Part model, mm, in its own coordinate system. A direction names the side the tool comes from. Round coordinates to 2 decimals unless told otherwise and drop trailing zeros. Write each loop counter-clockwise with the first axis right and the second up, starting at its lowest first coordinate (ties: lowest second). Pieces come first, ordered by that corner, then holes. Notation, with made-up numbers: M 26,72.5 L 42,72.5 A22 cw 42,96.5 Z; hole C 33.25,-37.75 d10. An arc over 180 degrees is marked long. Use a Markdown table: item, result. Add a question column.
1) Slice it at B-B on x = -7.5. Write the cut outline in (y, z), plus the area to 3 significant figures.
2) Two-plate mould, pull along Y, no slides. Class faces 1 (the face through (0, 2, -1)), 2 (the face through (-12.5, 5, -19)), 3 (the face through (0.2, 5.1, -19.5)): released by +Y, released by -Y, zero draft, split by the parting line, or undercut.
3) Wall check: probe 1 along Y at (x, z) = (0.35, -6); probe 2 along Y at (x, z) = (2.5, -22); probe 3 along X at (y, z) = (4.5, -4.25). Give the ranges that are in metal, low to high.
4) Slice it at A-A on z = -22. Write the cut outline in (x, y), plus the area to 3 significant figures.
5) Drop flat-ended pins along their axis: P1, Ø5, axis at x = -10, y = 5.5, coming from the +Z side; P2, Ø10, axis at x = -5, z = -10, coming from the +Y side; P3, Ø5, axis at y = 5, z = -6, coming from the -X side; P4, Ø3, axis at y = 3, z = -6, coming from the +X side. Give the stop position or say it passes through.
6) Slice it at D-D on z = -6. Write the cut outline in (x, y).
7) Slice it at C-C on y = 4.5. Write the cut outline in (x, z), plus the area to 3 significant figures.
8) Which spindle directions (+Z, -Z, +X, -X, +Y, -Y) get a long thin tool onto all of the face, cutting with end or side? Do faces 4 (the face through (0, 4.1, -4.8)), 5 (the face through (8, 5, -12)), 6 (the face through (-2.5, 3.8, -7.2)). Say none if no direction does.
```python
from build123d import *

# Parameters (mm, degrees)
BOSS_EXTRUDE1_DEPTH = 10
SKETCH2_R           = 2.5
SKETCH2_R_2         = 1.5
CUT_EXTRUDE1_DEPTH  = 39.13135193
FILLET1_R           = 5


with BuildPart() as part:
    # Sketch1 → Boss-Extrude1 (new body)
    with BuildSketch(Plane(origin=(0, 0, 0), x_dir=(1, 0, 0), z_dir=(0, 1, 0))):
        Polygon((2.5, 0), (-2.5, 0), (-2.5, 12), (-12.5, 12), (-12.5, 27), (12.5, 27), (12.5, 12), (2.5, 12), align=None)
    extrude(amount=BOSS_EXTRUDE1_DEPTH)

    # Sketch2 → Cut-Extrude1 (cut, through all)
    with BuildSketch(Plane(origin=(12.5, 0, 0), x_dir=(0, 0, -1), z_dir=(1, 0, 0))):
        with Locations((22, 5)):
            Circle(SKETCH2_R)
        with Locations((6, 5)):
            Circle(SKETCH2_R_2)
    extrude(amount=-CUT_EXTRUDE1_DEPTH, mode=Mode.SUBTRACT)

    # Fillet1
    fillet1_edges = [part.edges().sort_by_distance(p)[0] for p in [
        (0, 10, 0),
        (0, 0, 0),
    ]]
    fillet(fillet1_edges, radius=FILLET1_R - 0.0001)  # a hair under: the kernel refuses the full size


solid = part.part
```
Entries:
| question | item | result |
|---|---|---|
| 1 | outline | M 0,-27 L 10,-27 L 10,-12 L 0,-12 Z; hole C 5,-22 d5 |
| 1 | area | 130 mm^2 |
| 2 | face 1 | released by -Y |
| 2 | face 2 | zero draft |
| 2 | face 3 | undercut |
| 3 | probe 1 | y = 0 to 3.5, 6.5 to 10 |
| 3 | probe 2 | y = 0 to 2.5, 7.5 to 10 |
| 3 | probe 3 | x = -2.5 to 2.5 |
| 4 | outline | M -12.5,0 L 12.5,0 L 12.5,2.5 L -12.5,2.5 Z; M -12.5,7.5 L 12.5,7.5 L 12.5,10 L -12.5,10 Z |
| 4 | area | 125 mm^2 |
| 5 | P1 | stops at z = -12 |
| 5 | P2 | stops at y = 10 |
| 5 | P3 | stops at x = -2.5 |
| 5 | P4 | stops at x = 2.5 |
| 6 | outline | M -2.5,0 L 2.5,0 L 2.5,3.5 L -2.5,3.5 Z; M -2.5,6.5 L 2.5,6.5 L 2.5,10 L -2.5,10 Z |
| 7 | outline | M -12.5,-27 L 12.5,-27 L 12.5,-24.45 L -12.5,-24.45 Z; M -12.5,-19.55 L 12.5,-19.55 L 12.5,-12 L 2.5,-12 L 2.5,-7.41 L -2.5,-7.41 L -2.5,-12 L -12.5,-12 Z; M -2.5,-4.59 L 2.5,-4.59 L 2.5,-0.03 L -2.5,-0.03 Z |
| 7 | area | 298 mm^2 |
| 8 | face 4 | +X, -X |
| 8 | face 5 | +Z, +X, +Y, -Y |
| 8 | face 6 | +Z, -X, +Y, -Y |
